Check sheet for the modelled part. Datum: model origin and axes. Units: mm. A direction names the side the tool comes from. Coordinates: 2 decimals unless noted, no trailing zeros. Write each loop counter-clockwise with the first axis right and the second up, starting at its lowest first coordinate (ties: lowest second). Pieces come first, ordered by that corner, then holes. Notation, with made-up numbers: (-23, -29.5) -> (12, -29.5) arc R21 ccw to (12, -4.5) -> close; hole circle Ø10 at (-24.75, 22). An arc over 180 degrees is marked (long way). One line per item, written item: value. Start each with the question number.
1) Set-up check for faces 5 (the flat face through (32, 37, 125.066)), 6 (the flat face through (18.339, 4.5, 25.6)), 7 (the flat face through (-26.661, 4.5, 25.1)): record each of +Z, -Z, +X, -X, +Y, -Y from which the full face is reachable in a straight line by a thin tool's end or side.
2) Sectioned sample at D-D on y = 20.5. Enter the section's corners in (x, z).
3) Draft check along Y on faces 1 (the flat face through (32, 43.4, 129)), 2 (the flat face through (-5, 12, 10.6)), 3 (the flat face through (45.05, 37, 129)), 4 (the flat face through (32, 17, 129.066)). Enter one of: +Y half, -Y half, draft (parallel to the pull), parting line (faces both ways), or undercut.
4) Scan lines: line 1 along X through (y, z) = (3, 75.5); line 2 along Y through (x, z) = (-14.5, 120); line 3 along Z through (x, y) = (-28, 38). Record each from-to range of solid material in increasing order. Write a range as [from, to].
5) Sectioned sample at C-C on x = 38.5. Enter the section's corners in (y, z).
6) Sectioned sample at A-A on y = 36. Enter the section's corners in (x, z).
7) Gauge pin test, flat ends, axial feed: P1, Ø3, axis at x = -6, z = 8, coming from the +Y side; P2, Ø8, axis at x = -18, y = 14, coming from the -Z side; P3, Ø14.5, axis at x = -33.5, y = 39.5, coming from the -Z side; P4, Ø1.3, axis at x = -12, z = 87.07, coming from the -Y side. Record the tip position at first contact, or that the pin passes through.
8) Sectioned sample at B-B on z = 76. Enter the section's corners in (x, y).
```python
from build123d import *

# Parameters (mm, degrees)
SUPERFICIE_DEITADA_W     = 45
SUPERFICIE_DEITADA_H     = 35.5
BOSS_EXTRUDE1_DEPTH      = 4
SUPERFICIE_DEITADA_4_W   = 45
SUPERFICIE_DEITADA_4_H   = 8
SUPERFICIE_DEITADA_4_H_2 = 19.5
BOSS_EXTRUDE2_DEPTH      = 15
SUPERFICIE_DEITADA_5_W   = 12
SUPERFICIE_DEITADA_5_H   = 35
SUPERFICIE_DEITADA_5_W_2 = 24
SUPERFICIE_DEITADA_5_H_2 = 40
SUPERFICIE_DEITADA_5_R   = 1.1
BOSS_EXTRUDE3_DEPTH      = 2
SUPERFICIE_DEITADA_6_W   = 25
SUPERFICIE_DEITADA_6_H   = 4
BOSS_EXTRUDE4_DEPTH      = 30
SUPERFICIE_DEITADA_7_W   = 25
SUPERFICIE_DEITADA_7_H   = 4
BOSS_EXTRUDE5_DEPTH      = 30
SUPERFICIE_VERTICAL_R    = 1.5
CUT_EXTRUDE1_DEPTH       = 200.4
CUT_EXTRUDE2_DEPTH       = 200.4
SKETCH5_W                = 8
SKETCH5_H                = 2
CUT_EXTRUDE3_DEPTH       = 8
CUT_EXTRUDE4_DEPTH       = 7
CUT_EXTRUDE4_DEPTH_BACK  = 3
SKETCH6_R                = 1.1
SKETCH8_W                = 8
SKETCH8_H                = 2
CUT_EXTRUDE5_DEPTH       = 8
CUT_EXTRUDE6_DEPTH       = 15
CUT_EXTRUDE6_DEPTH_BACK  = 3
SKETCH9_R                = 1.1
SKETCH11_W               = 25.05
SKETCH11_H               = 8
BOSS_EXTRUDE6_DEPTH      = 13.4
SKETCH12_W               = 25
SKETCH12_H               = 8
BOSS_EXTRUDE7_DEPTH      = 13.4


with BuildPart() as part:
    # Superficie_Deitada → Boss-Extrude1 (new body)
    with BuildSketch(Plane(origin=(0, 0, 0), x_dir=(1, 0, 0), z_dir=(0, 1, 0))):
        Polygon((-20, -129.066204139), (-20, -133.066204139), (20, -133.066204139), (20, -129.066204139), (45, -129.066204139), (45, 54.433795861), (-45, 54.433795861), (-45, -129.066204139), align=None)
        with Locations((-4.160854438, -25.316204139)):
            Rectangle(SUPERFICIE_DEITADA_W, SUPERFICIE_DEITADA_H, mode=Mode.SUBTRACT)
        Polygon((-43, -48.066204139), (-31, -48.066204139), (-31, -83.066204139), (-7, -83.066204139), (-7, -123.066204139), (-43, -123.066204139), align=None, mode=Mode.SUBTRACT)
    extrude(amount=BOSS_EXTRUDE1_DEPTH)

    # Superficie_Deitada<4> → Boss-Extrude2 (add)
    with BuildSketch(Plane(origin=(0, 0, 0), x_dir=(1, 0, 0), z_dir=(0, 1, 0))):
        with Locations((-4.160854438, -11.566204139)):
            Rectangle(SUPERFICIE_DEITADA_4_W, SUPERFICIE_DEITADA_4_H)
        with Locations((-4.160854438, -25.316204139)):
            Rectangle(SUPERFICIE_DEITADA_4_W, SUPERFICIE_DEITADA_4_H_2)
        with Locations((-4.160854438, -39.066204139)):
            Rectangle(SUPERFICIE_DEITADA_4_W, SUPERFICIE_DEITADA_4_H)
    extrude(amount=BOSS_EXTRUDE2_DEPTH)

    # Superficie_Deitada<5> → Boss-Extrude3 (add)
    # profile 1 of 3: a face of its own
    with BuildSketch(Plane(origin=(0, 0, 0), x_dir=(1, 0, 0), z_dir=(0, 1, 0))):
        with Locations((-37, -65.566204139)):
            Rectangle(SUPERFICIE_DEITADA_5_W, SUPERFICIE_DEITADA_5_H)
    # profile 2 of 3: a face of its own
    with BuildSketch(Plane(origin=(0, 0, 0), x_dir=(1, 0, 0), z_dir=(0, 1, 0))):
        with Locations((-19, -103.066204139)):
            Rectangle(SUPERFICIE_DEITADA_5_W_2, SUPERFICIE_DEITADA_5_H_2)
        with Locations(Location((-18, -93.066204139, 0), (0, 0, 270))):
            Circle(SUPERFICIE_DEITADA_5_R, mode=Mode.SUBTRACT)
        with Locations(Location((-18, -87.066204139, 0), (0, 0, 270))):
            Circle(SUPERFICIE_DEITADA_5_R, mode=Mode.SUBTRACT)
        with Locations(Location((-12, -93.066204139, 0), (0, 0, 270))):
            Circle(SUPERFICIE_DEITADA_5_R, mode=Mode.SUBTRACT)
        with Locations(Location((-12, -87.066204139, 0), (0, 0, 270))):
            Circle(SUPERFICIE_DEITADA_5_R, mode=Mode.SUBTRACT)
    # profile 3 of 3: a face of its own
    with BuildSketch(Plane(origin=(0, 0, 0), x_dir=(1, 0, 0), z_dir=(0, 1, 0))):
        with Locations((-37, -103.066204139)):
            Rectangle(SUPERFICIE_DEITADA_5_W, SUPERFICIE_DEITADA_5_H_2)
    extrude(amount=BOSS_EXTRUDE3_DEPTH)

    # Superficie_Deitada<6> → Boss-Extrude4 (add)
    with BuildSketch(Plane(origin=(0, 0, 0), x_dir=(1, 0, 0), z_dir=(0, 1, 0))):
        with Locations((32.5, -131.066204139)):
            Rectangle(SUPERFICIE_DEITADA_6_W, SUPERFICIE_DEITADA_6_H)
    extrude(amount=BOSS_EXTRUDE4_DEPTH)

    # Superficie_Deitada<7> → Boss-Extrude5 (add)
    with BuildSketch(Plane(origin=(0, 0, 0), x_dir=(1, 0, 0), z_dir=(0, 1, 0))):
        with Locations((-32.5, -131.066204139)):
            Rectangle(SUPERFICIE_DEITADA_7_W, SUPERFICIE_DEITADA_7_H)
    extrude(amount=BOSS_EXTRUDE5_DEPTH)

    # Superficie_vertical → Cut-Extrude1 (cut)
    with BuildSketch(Plane.XY):
        with Locations(Location((32.5, 25, 0), (0, 0, 180))):
            Circle(SUPERFICIE_VERTICAL_R)
        with Locations(Location((-35, 25, 0), (0, 0, 180))):
            Circle(SUPERFICIE_VERTICAL_R)
    extrude(amount=CUT_EXTRUDE1_DEPTH, mode=Mode.SUBTRACT)

    # Sketch4 → Cut-Extrude2 (cut)
    with BuildSketch(Plane.ZY.offset(26.660854438)):
        with BuildLine():
            ThreePointArc((35.316204139, 15), (25.316204139, 25), (15.316204139, 15))
            Line((15.316204139, 15), (15.566204139, 15))
            Line((15.566204139, 15), (35.066204139, 15))
            Line((35.066204139, 15), (35.316204139, 15))
        make_face()
        with BuildLine():
            Line((15.566204139, 15), (15.316204139, 15))
            ThreePointArc((15.316204139, 15), (25.316204139, 5), (35.316204139, 15))
            Line((35.316204139, 15), (35.066204139, 15))
            Line((35.066204139, 15), (15.566204139, 15))
        make_face()
    extrude(amount=-CUT_EXTRUDE2_DEPTH, mode=Mode.SUBTRACT)

    # Sketch5 → Cut-Extrude3 (cut)
    with BuildSketch(Plane(origin=(0, 0, 7.566204139), x_dir=(-1, 0, 0), z_dir=(0, 0, -1))):
        with Locations((4.160854438, 11)):
            Rectangle(SKETCH5_W, SKETCH5_H)
    extrude(amount=-CUT_EXTRUDE3_DEPTH, mode=Mode.SUBTRACT)

    # Sketch6 → Cut-Extrude4 (cut, two sides: drawn at the far end of the back side and taken through both)
    with BuildSketch(Plane(origin=(0, 10, 0), x_dir=(1, 0, 0), z_dir=(0, 1, 0)).offset(-CUT_EXTRUDE4_DEPTH_BACK)):
        with Locations(Location((-4.160854438, -11.566204139, 0), (0, 0, 270))):
            Circle(SKETCH6_R)
    extrude(amount=CUT_EXTRUDE4_DEPTH + CUT_EXTRUDE4_DEPTH_BACK, mode=Mode.SUBTRACT)

    # Sketch8 → Cut-Extrude5 (cut)
    with BuildSketch(Plane.XY.offset(43.066204139)):
        with Locations((-4.160854438, 10)):
            Rectangle(SKETCH8_W, SKETCH8_H)
    extrude(amount=-CUT_EXTRUDE5_DEPTH, mode=Mode.SUBTRACT)

    # Sketch9 → Cut-Extrude6 (cut, two sides: drawn at the far end of the back side and taken through both)
    with BuildSketch(Plane(origin=(0, 9, 0), x_dir=(1, 0, 0), z_dir=(0, 1, 0)).offset(-CUT_EXTRUDE6_DEPTH_BACK)):
        with Locations(Location((-4.160854438, -39.066204139, 0), (0, 0, 270))):
            Circle(SKETCH9_R)
    extrude(amount=CUT_EXTRUDE6_DEPTH + CUT_EXTRUDE6_DEPTH_BACK, mode=Mode.SUBTRACT)

    # Sketch11 → Boss-Extrude6 (add)
    with BuildSketch(Plane(origin=(0, 30, 0), x_dir=(1, 0, 0), z_dir=(0, 1, 0))):
        with Locations((32.525, -129.066204139)):
            Rectangle(SKETCH11_W, SKETCH11_H)
    extrude(amount=BOSS_EXTRUDE6_DEPTH)

    # Sketch12 → Boss-Extrude7 (add)
    with BuildSketch(Plane(origin=(0, 30, 0), x_dir=(1, 0, 0), z_dir=(0, 1, 0))):
        with Locations((-32.5, -129.066204139)):
            Rectangle(SKETCH12_W, SKETCH12_H)
    extrude(amount=BOSS_EXTRUDE7_DEPTH)


solid = part.part
```
Answers:
1. face 5: -Z, +X, -X, +Y
1. face 6: +Z, -Z, +X, +Y
1. face 7: -Z, -X, +Y
2. outline: (-45, 129.07) -> (-20, 129.07) -> (-20, 133.07) -> (-45, 133.07) -> close; (20, 129.07) -> (45, 129.07) -> (45, 133.07) -> (20, 133.07) -> close
3. face 1: +Y half
3. face 2: undercut
3. face 3: draft
3. face 4: undercut
4. line 1: x = [-45, -43], [-31, 45]
4. line 2: y = [0, 2]
4. line 3: z = [125.07, 133.07]
5. outline: (0, -54.43) -> (4, -54.43) -> (4, 129.07) -> (30, 129.07) -> (30, 125.07) -> (43.4, 125.07) -> (43.4, 133.07) -> (0, 133.07) -> close
6. outline: (-45, 125.07) -> (-20, 125.07) -> (-20, 133.07) -> (-45, 133.07) -> close; (20, 125.07) -> (45.05, 125.07) -> (45.05, 133.07) -> (20, 133.07) -> close
7. P1: stops at y = 15
7. P2: stops at z = 7.57
7. P3: stops at z = 125.07
7. P4: passes through
8. outline: (-45, 0) -> (45, 0) -> (45, 4) -> (-31, 4) -> (-31, 2) -> (-43, 2) -> (-43, 4) -> (-45, 4) -> close
